For this review, take the finished solid that the model builds, in its own axes (mm). Give positions to 0.01 mm unless a question says otherwise; leave off trailing zeros. Order: outer loops, then holes, each group sorted by start corner. A loop starts at its lowest first (then second) coordinate and runs counter-clockwise, first axis right, second up. Notation, with made-up numbers: (-16.5, -17.75) -> (35.5, -17.75) arc R17 cw to (35.5, -6.75) -> close; hole circle Ø10 at (-12.5, -10.75). An arc over 180 degrees is marked (long way). One line per item, written item: value. Start each with the question number.
from build123d import *

# Parameters (mm, degrees)
SKETCH1_W           = 300
SKETCH1_H           = 250
SKETCH1_R           = 2
BOSS_EXTRUDE1_DEPTH = 5
SKETCH2_W           = 140
SKETCH2_H           = 185
CUT_EXTRUDE1_DEPTH  = 196.320249846
FILLET1_R           = 20


with BuildPart() as part:
    # Sketch1 → Boss-Extrude1 (new body)
    with BuildSketch(Plane(origin=(0, 0, 0), x_dir=(1, 0, 0), z_dir=(0, 1, 0))):
        Rectangle(SKETCH1_W, SKETCH1_H)
        with Locations(Location((-140, -115, 0), (0, 0, 270))):
            Circle(SKETCH1_R, mode=Mode.SUBTRACT)
        with Locations(Location((-140, 115, 0), (0, 0, 90))):
            Circle(SKETCH1_R, mode=Mode.SUBTRACT)
        with Locations(Location((140, -115, 0), (0, 0, 90))):
            Circle(SKETCH1_R, mode=Mode.SUBTRACT)
        with Locations(Location((140, 115, 0), (0, 0, 270))):
            Circle(SKETCH1_R, mode=Mode.SUBTRACT)
    extrude(amount=BOSS_EXTRUDE1_DEPTH)

    # Sketch2 → Cut-Extrude1 (cut, through all)
    with BuildSketch(Plane(origin=(0, 5, 0), x_dir=(1, 0, 0), z_dir=(0, 1, 0))):
        with Locations((0, 32.5)):
            Rectangle(SKETCH2_W, SKETCH2_H)
    extrude(amount=-CUT_EXTRUDE1_DEPTH, mode=Mode.SUBTRACT)

    # Fillet1
    fillet1_edges = [part.edges().sort_by_distance(p)[0] for p in [
        (-70, 2.5, 60),
        (70, 2.5, 60),
    ]]
    fillet(fillet1_edges, radius=FILLET1_R)


solid = part.part
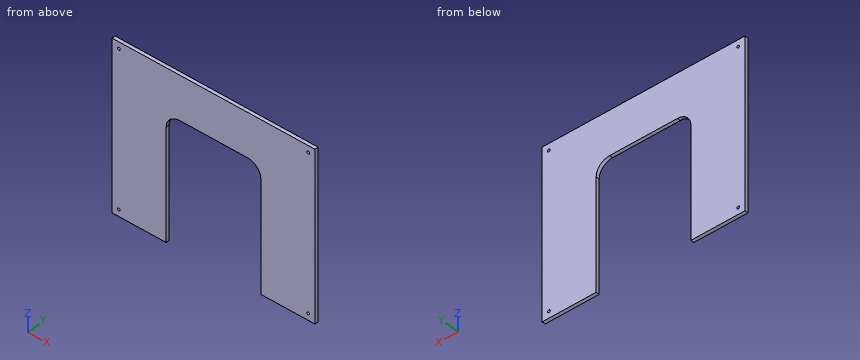
Q1. Take a section at A-A (z = -35). State the section outline as (x, y) points.
Q2. For line 1 along X through (y, z) = (1.5, 115); line 2 along Z through (x, y) = (140, 1.3); line 3 along X through (y, z) = (1.7, -115), list the stretches that pass through material, from the lowest coordinate up.
Q3. Take a section at B-B (y = 2.15). State the section outline as (x, z) points, and give its area (3 significant figures).
Q4. Take a section at C-C (x = -19). State the section outline as (y, z) points.
Answers below:
1. outline: (-150, 0) -> (-70, 0) -> (-70, 5) -> (-150, 5) -> close; (70, 0) -> (150, 0) -> (150, 5) -> (70, 5) -> close
2. line 1: x = -150 to -142, -138 to 138, 142 to 150
2. line 2: z = -125 to -117, -113 to 113, 117 to 125
2. line 3: x = -150 to -142, -138 to -70, 70 to 138, 142 to 150
3. outline: (-150, -125) -> (-70, -125) -> (-70, 40) arc R20 cw to (-50, 60) -> (50, 60) arc R20 cw to (70, 40) -> (70, -125) -> (150, -125) -> (150, 125) -> (-150, 125) -> close; hole circle Ø4 at (-140, -115); hole circle Ø4 at (-140, 115); hole circle Ø4 at (140, -115); hole circle Ø4 at (140, 115)
3. area: 49,200 mm²
4. outline: (0, 60) -> (5, 60) -> (5, 125) -> (0, 125) -> close
